Autodesk Inventor part; units mm, degrees
ref_plane "YZ Plane" through (0, 0, 0) normal (1, 0, 0) x (0, 1, 0)
ref_plane "XZ Plane" through (0, 0, 0) normal (0, 1, 0) x (-1, 0, 0)
ref_plane "XY Plane" through (0, 0, 0) normal (0, 0, 1) x (1, 0, 0)
sketch "Sketch1" plane through (0, 0, 0) normal (0, 1, 0) x (-1, 0, 0)
  line L0 (-5, -3) -> (5, -3)
  line L1 (5, -3) -> (5, 3)
  line L2 (5, 3) -> (-5, 3)
  line L3 (-5, 3) -> (-5, -3)
  line L4 (-5, -3) -> (5, 3) construction
  line L5 (5, -3) -> (-5, 3) construction
  line L6 (2.8, 3) -> (2.8, -3)
  line L7 (-2.8, -3) -> (-2.8, 3)
  line L8 (-2.8, 0) -> (2.8, 0) construction
  circle A0 centre (0, 0) radius 2
  dimension "d0" = 10
  dimension "d1" = 6
  dimension "d5" = 5.6
  dimension "d11" = 4
extrude "Extrusion1" add sketch "Sketch1" along normal blind 4.2
extrude "Extrusion2" cut sketch "Sketch1" along normal blind 0.9 contours L3 L2 L7 L0 | L6 L2 L1 L0
chamfer "Chamfer1" distance 2 angle 45 2 edges at (-5, 4.2, 0) (5, 4.2, 0)
fillet "Fillet1" radius 1.5 4 edges at (-3, 4.2, 0) (3, 4.2, 0) (-5, 2.2, 0) (5, 2.2, 0)
properties part number "M4 T-Slot Nut"
For this review, take the finished solid that the model builds, in its own axes (mm). A direction names the side the tool comes from. Coordinates: 2 decimals unless noted, no trailing zeros. Write each loop counter-clockwise with the first axis right and the second up, starting at its lowest first coordinate (ties: lowest second). Pieces come first, ordered by that corner, then holes. Notation, with made-up numbers: (30, 67.5) - (67, 67.5) arc R24 ccw to (67, 104.5) - close; hole circle Ø1 at (-22.5, -24.5). An arc over 180 degrees is marked (long way). Put each result on its own line as item: value.
1. Add section B-B, the plane x = 0. Give the boundary of the cut face in (y, z).
Values found:
outline: (0, -3) - (4.2, -3) - (4.2, -2) - (0, -2) - close; (0, 2) - (4.2, 2) - (4.2, 3) - (0, 3) - close
2. Add section C-C, the plane y = 1.4. Give the boundary of the cut face in (x, z).
Values found:
outline: (-5, -3) - (5, -3) - (5, 3) - (-5, 3) - close; hole circle Ø4 at (0, 0)
3. Wall thickness on probe 1 along Z at (x, y) = (0, 2.6); probe 2 along X at (y, z) = (1.6, 0.1); probe 3 along Z at (x, y) = (0.5, 3.9): over which ranges is each line inside the solid? List them lowest first.
Values found:
probe 1: -3 to -2, 2 to 3
probe 2: -5 to -2, 2 to 5
probe 3: -3 to -1.94, 1.94 to 3
4. Mouldability with a two-part tool opening along Z and no side actions: class faces 1 (the flat face through (0, 2, -3)), 2 (the cylindrical face through (2.945, 4.089, -0.042)), 3 (the cylindrical face through (0, 2, 2)) as released by +Z, released by -Z, zero draft, split by the parting line, or undercut.
Values found:
face 1: released by -Z
face 2: zero draft
face 3: undercut
5. Add section A-A, the plane z = 0. Give the boundary of the cut face in (x, y), then the cut area to 3 significant figures.
Values found:
outline: (-5, 0.9) - (-2.8, 0.9) - (-2.8, 0) - (-2, 0) - (-2, 4.2) - (-2.38, 4.2) arc R1.5 ccw to (-3.44, 3.76) - (-4.56, 2.64) arc R1.5 ccw to (-5, 1.58) - close; (2, 0) - (2.8, 0) - (2.8, 0.9) - (5, 0.9) - (5, 1.58) arc R1.5 ccw to (4.56, 2.64) - (3.44, 3.76) arc R1.5 ccw to (2.38, 4.2) - (2, 4.2) - close
area: 17.0 mm²
6. Machinability: for faces 4 (the flat face through (4, 3.2, 0)), 5 (the flat face through (-2.8, 0.4, 0)), 6 (the flat face through (2.8, 0.4, 0)), which of the approach directions +Z, -Z, +X, -X, +Y, -Y give a long, thin tool a straight path to every point of the face, cutting with its end or side? Answer none if there is none.
Values found:
face 4: +Z, -Z, +X, +Y
face 5: +Z, -Z, -X, -Y
face 6: +Z, -Z, +X, -Y
7. Add section D-D, the plane z = 2.25. Give the boundary of the cut face in (x, y).
Values found:
outline: (-5, 0.9) - (-2.8, 0.9) - (-2.8, 0) - (2.8, 0) - (2.8, 0.9) - (5, 0.9) - (5, 1.58) arc R1.5 ccw to (4.56, 2.64) - (3.44, 3.76) arc R1.5 ccw to (2.38, 4.2) - (-2.38, 4.2) arc R1.5 ccw to (-3.44, 3.76) - (-4.56, 2.64) arc R1.5 ccw to (-5, 1.58) - close
